Check sheet for the drawn part. Datum: minimum x, y, z corner. Units: mm. A direction names the side the tool comes from. Coordinates: 2 decimals unless noted, no trailing zeros. Loops run counter-clockwise (first coordinate to the right, second up) from the corner with the lowest first, then second, coordinate; pieces in that order, holes last.
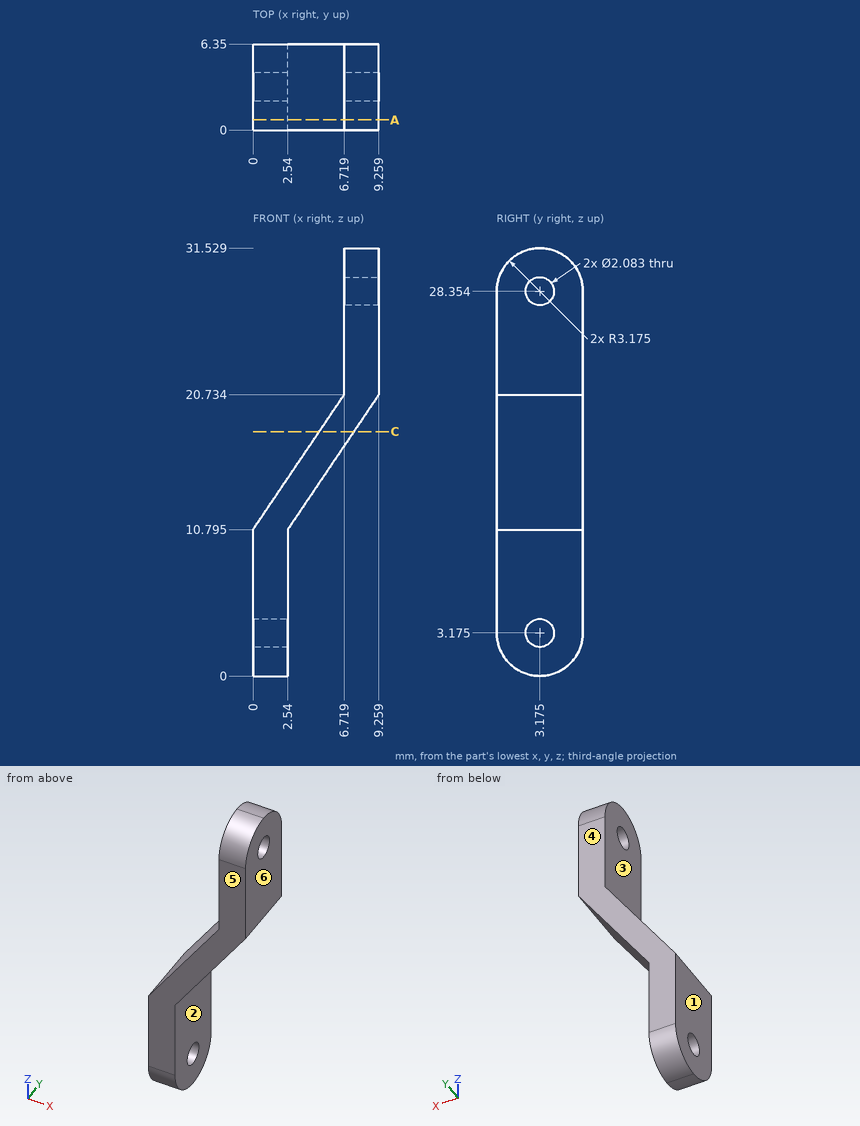
(1) Gauge pin test, flat ends, axial feed: pin 1 Ø3 at (y, z) = (3.5, 27) entering from -X; pin 2 Ø2.5 at (y, z) = (3.175, 3.175) entering from +X; pin 3 Ø1.5 at (x, y) = (5.5, 4) entering from +Z; pin 4 Ø1.2 at (y, z) = (3.18, 28.35) entering from +X. Record the tip position at first contact, or that the pin passes through.
Findings:
pin 1: stops at x = 6.72
pin 2: stops at x = 2.54
pin 3: stops at z = 20.04
pin 4: passes through
(2) Sectioned sample at A-A on y = 0.75. Record the cut outline in (x, z) (1 decimal).
Findings:
outline: (0, 1.1) - (2.5, 1.1) - (2.5, 10.8) - (9.3, 20.7) - (9.3, 30.4) - (6.7, 30.4) - (6.7, 20.7) - (0, 10.8) - close
(3) Draft check along Y on the marked faces 4, 5 and 6. Enter one of: +Y half, -Y half, draft (parallel to the pull), parting line (faces both ways), or undercut.
Findings:
face 4: +Y half
face 5: -Y half
face 6: draft
(4) Sectioned sample at C-C on z = 18. Record the cut outline in (x, y).
Findings:
outline: (4.87, 0) - (7.41, 0) - (7.41, 6.35) - (4.87, 6.35) - close
(5) Scan lines: L1, parallel to X at y = 2, z = 22; L2, parallel to Z at x = 2.25, y = 2.5 (1 decimal); L3, parallel to X at y = 1.5, z = 8.5. Record each from-to range of solid material in increasing order.
Findings:
L1: x = 6.72 to 9.26
L2: z = 0.1 to 2.4, 4 to 14.1
L3: x = 0 to 2.54
(6) Access from +Z, -Z, +X, -X, +Y, -Y to the whole of each face (thin tool, end or side, straight path). Record for the marked faces 1, 2 and 3.
Findings:
face 1: +Z, -Z, -X, +Y, -Y
face 2: -Z, +X, +Y, -Y
face 3: +Z, -X, +Y, -Y
